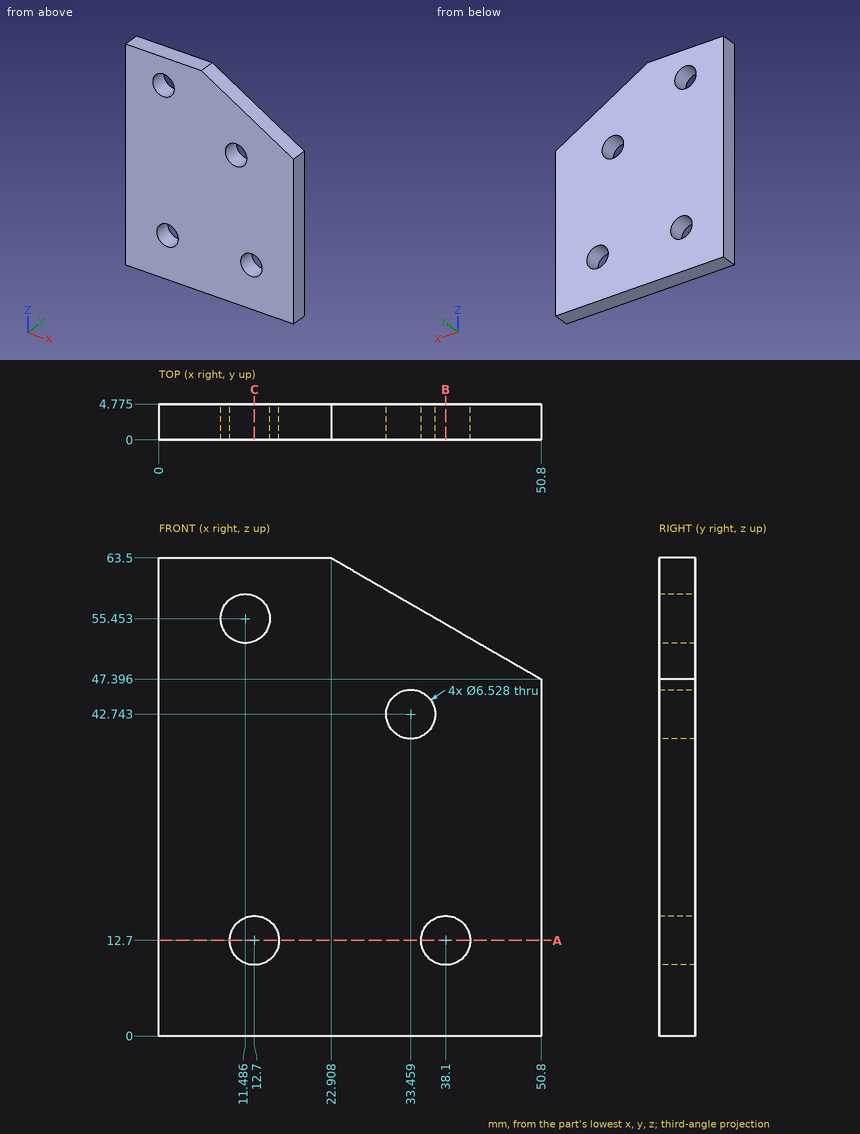
Answer from the drawing. Dimensions are ordinates in mm from the lowest x, y and z of the part. Coordinates: 2 decimals unless noted, no trailing zeros. Write each loop counter-clockwise with the first axis right and the second up, starting at its lowest first coordinate (ties: lowest second). Pieces come first, ordered by that corner, then holes. Notation, with made-up numbers: (-35.5, -36.5) - (15.5, -36.5) arc R25 cw to (15.5, -22.5) - close; hole circle Ø1 at (-24.5, -7). An arc over 180 degrees is marked (long way). Return JSON: item names as keys, results as strings. Group by question number.
Q1. The part is cut by section A-A on z = 12.7. Write down the section's boundary in (x, y) (1 decimal).
Q2. The part is cut by section C-C on x = 12.7. Write down the section's boundary in (y, z) (1 decimal).
Q3. Find the intervals of material crossed by line 1 along X through (y, z) = (1.8, 12.7); line 2 along Z through (x, y) = (12, 4.35); line 3 along Z through (x, y) = (38.1, 1.15) (1 decimal), in increasing order. Write a range as [from, to].
Q4. A flat-ended cylindrical pin translates along its axis: pin 1 Ø1.5 at (x, y) = (42.5, 3) entering from +Z. Find the tip coordinate at first contact, or state that the pin passes through.
Q5. The part is cut by section B-B on x = 38.1. Write down the section's boundary in (y, z) (1 decimal).
Evaluation:
{
 "1": {"outline": "(0, 0) - (9.4, 0) - (9.4, 4.8) - (0, 4.8) - close; (16, 0) - (34.8, 0) - (34.8, 4.8) - (16, 4.8) - close; (41.4, 0) - (50.8, 0) - (50.8, 4.8) - (41.4, 4.8) - close"},
 "2": {"outline": "(0, 0) - (4.8, 0) - (4.8, 9.4) - (0, 9.4) - close; (0, 16) - (4.8, 16) - (4.8, 52.4) - (0, 52.4) - close; (0, 58.5) - (4.8, 58.5) - (4.8, 63.5) - (0, 63.5) - close"},
 "3": {"line 1": "x = [0, 9.44], [15.96, 34.84], [41.36, 50.8]", "line 2": "z = [0, 9.51], [15.89, 52.23], [58.68, 63.5]", "line 3": "z = [0, 9.4], [16, 54.7]"},
 "4": {"pin 1": "stops at z = 52.62"},
 "5": {"outline": "(0, 0) - (4.8, 0) - (4.8, 9.4) - (0, 9.4) - close; (0, 16) - (4.8, 16) - (4.8, 54.7) - (0, 54.7) - close"}
}
